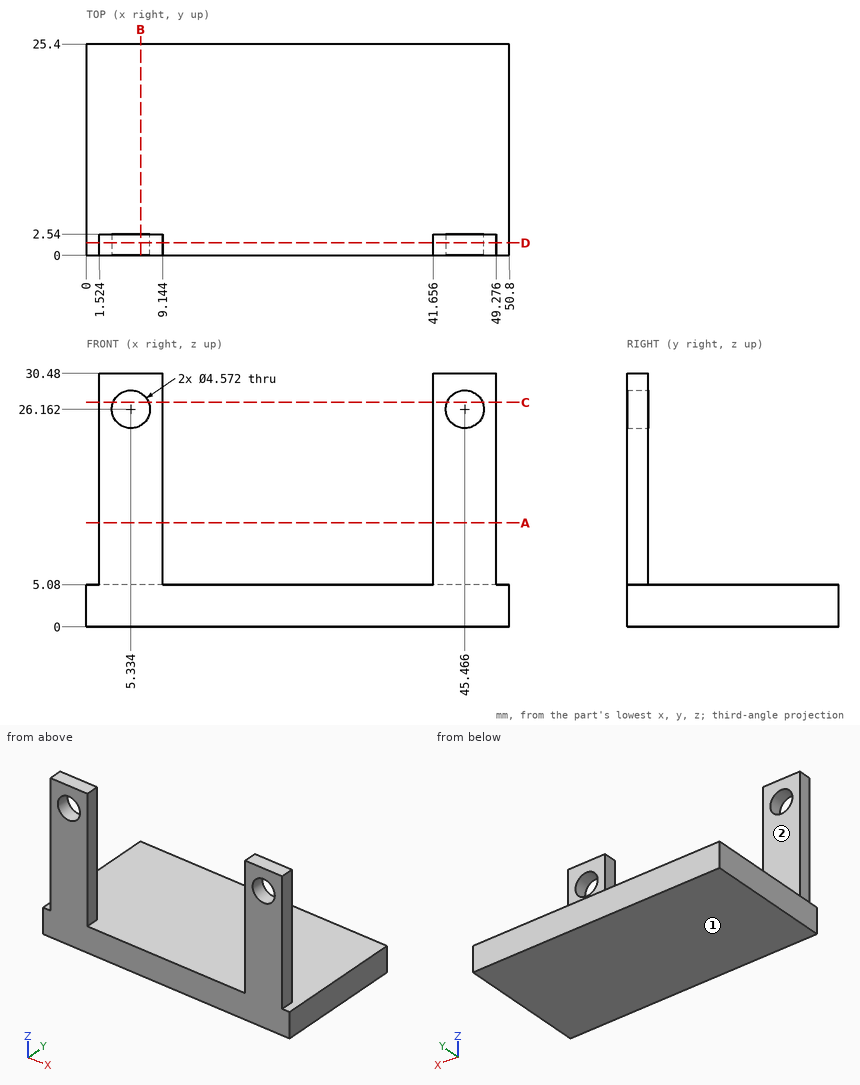
Here's the drawing with two shaded views (mm, measured from the low corner). I have some questions. A direction names the side the tool comes from. Round coordinates to 2 decimals unless told otherwise and drop trailing zeros. Loops run counter-clockwise (first coordinate to the right, second up) from the corner with the lowest first, then second, coordinate; pieces in that order, holes last. Notation, with made-up numbers: M -36.5,7.25 L -15.5,7.25 A20 cw -15.5,17.25 Z; hole C 29,36.5 d4. An arc over 180 degrees is marked long. Answer as CSV lines item,"result".
1) Which directions (+Z, -Z, +X, -X, +Y, -Y) give clear straight access to the entire face, cutting with the end or side of a thin tool? Please do the marked faces 1 and 2.
From the geometry:
face 1,"-Z, +X, -X, +Y, -Y"
face 2,"+Z, +X, -X, +Y"
2) For pin 1 Ø3 at (x, y) = (9, 5) entering from +Z; pin 2 Ø4 at (x, z) = (46.5, 18) entering from +Y; pin 3 Ø3 at (y, z) = (0.5, 22.5) entering from -X, each with a flat end and sliding along its axis, tell me the tip position at first contact or that it passes through.
From the geometry:
pin 1,"z = 5.08"
pin 2,"y = 2.54"
pin 3,"x = 1.52"
3) Imagine slicing it at D-D on y = 1.5. List the corners of the cut face in (x, z) for me, and give its area (3 significant figures).
From the geometry:
outline,"M 0,0 L 50.8,0 L 50.8,5.08 L 49.28,5.08 L 49.28,30.48 L 41.66,30.48 L 41.66,5.08 L 9.14,5.08 L 9.14,30.48 L 1.52,30.48 L 1.52,5.08 L 0,5.08 Z; hole C 5.33,26.16 d4.57; hole C 45.47,26.16 d4.57"
area,"612 mm^2"
4) Imagine slicing it at B-B on x = 6.5. List the corners of the cut face in (y, z) for me.
From the geometry:
outline,"M 0,0 L 25.4,0 L 25.4,5.08 L 2.54,5.08 L 2.54,24.2 L 0,24.2 Z; M 0,28.13 L 2.54,28.13 L 2.54,30.48 L 0,30.48 Z"
5) Imagine slicing it at C-C on z = 27. List the corners of the cut face in (x, y) for me, and give its area (3 significant figures).
From the geometry:
outline,"M 1.52,0 L 3.21,0 L 3.21,2.54 L 1.52,2.54 Z; M 7.46,0 L 9.14,0 L 9.14,2.54 L 7.46,2.54 Z; M 41.66,0 L 43.34,0 L 43.34,2.54 L 41.66,2.54 Z; M 47.59,0 L 49.28,0 L 49.28,2.54 L 47.59,2.54 Z"
area,"17.1 mm^2"
6) Imagine slicing it at A-A on z = 12.5. List the corners of the cut face in (x, y) for me.
From the geometry:
outline,"M 1.52,0 L 9.14,0 L 9.14,2.54 L 1.52,2.54 Z; M 41.66,0 L 49.28,0 L 49.28,2.54 L 41.66,2.54 Z"
7) If I drill on probe 1 along Z at (x, y) = (17.5, 22); probe 2 along Y at (x, z) = (42, 25); probe 3 along X at (y, z) = (2, 27), over which ranges is the centre line in solid material (lowest first)?
From the geometry:
probe 1,"0 to 5.08"
probe 2,"0 to 2.54"
probe 3,"1.52 to 3.21, 7.46 to 9.14, 41.66 to 43.34, 47.59 to 49.28"
